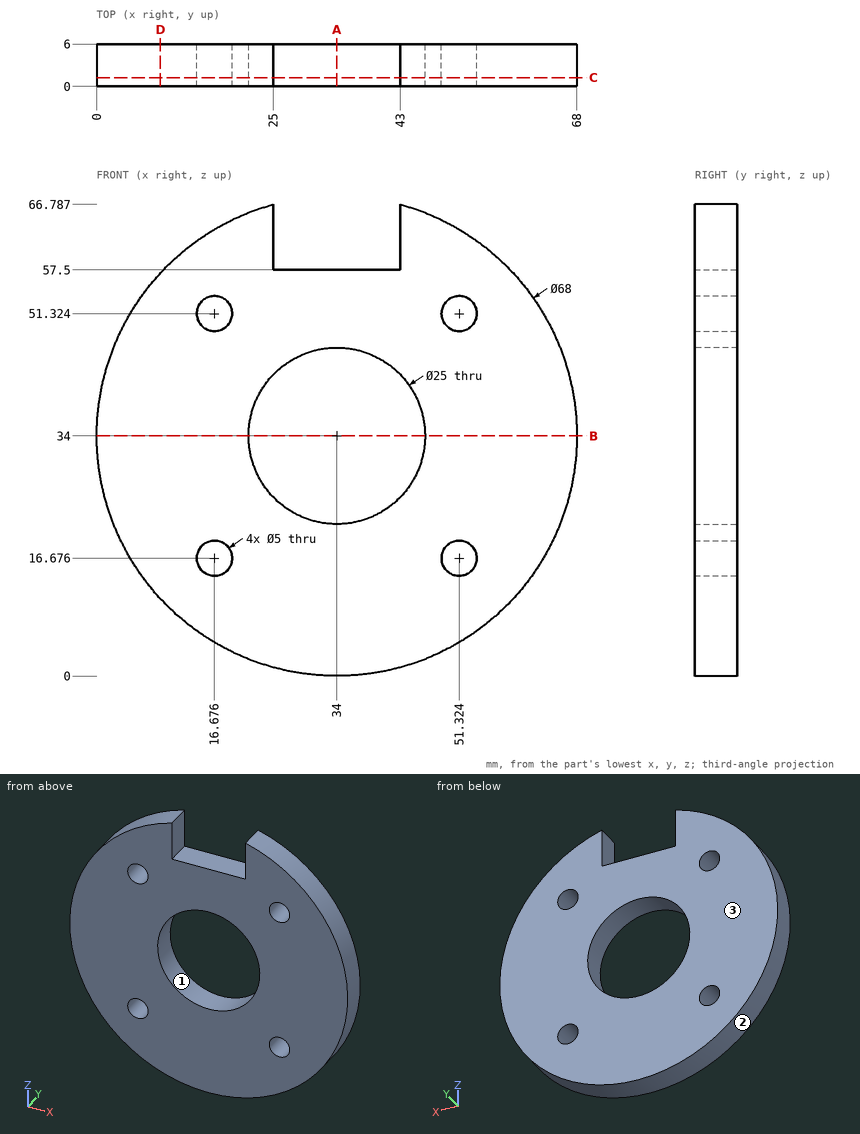
Check sheet for the drawn part. Datum: minimum x, y, z corner. Units: mm. Coordinates: 2 decimals unless noted, no trailing zeros. Order: outer loops, then holes, each group sorted by start corner. A loop starts at its lowest first (then second) coordinate and runs counter-clockwise, first axis right, second up. Notation, with made-up numbers: M 75,8 L 125,8 A10 cw 125,14 Z; hole C 9,28 d8. An arc over 180 degrees is marked long. One line per question, with ' | ' between items. Start each with the question number.
Item 1: Sectioned sample at A-A on x = 34. Record the cut outline in (y, z), and give its area (3 significant figures).
Item 2: Mould release check, pull along Z, two halves, no side actions. Record for the marked faces 1, 2 and 3: pulls with the +Z half, pulls with the -Z half, needs draft (parallel to the pull), parting line crosses it, or undercut.
Item 3: Sectioned sample at D-D on x = 9. Record the cut outline in (y, z).
Item 4: Material ranges on line 1 (Z direction, x = 18, y = 4.25) (1 decimal); line 2 (X direction, y = 2.7, z = 14.5) (1 decimal); line 3 (X direction, y = 5.4, z = 51) (1 decimal), recorded low to high.
Item 5: Sectioned sample at B-B on z = 34. Record the cut outline in (x, y).
Item 6: Gauge pin test, flat end, axial feed: P1, Ø1.8, axis at x = 35, y = 3.5, coming from the +Z side. Record the tip position at first contact, or that the pin passes through.
Item 7: Sectioned sample at C-C on y = 1.25. Record the cut outline in (x, z), and give its area (3 significant figures).
Answer below:
1) outline: M 0,0 L 6,0 L 6,21.5 L 0,21.5 Z; M 0,46.5 L 6,46.5 L 6,57.5 L 0,57.5 Z | area: 195 mm^2
2) face 1: undercut | face 2: parting line crosses it | face 3: needs draft
3) outline: M 0,10.96 L 6,10.96 L 6,57.04 L 0,57.04 Z
4) line 1: z = 4 to 14.6, 18.8 to 49.2, 53.4 to 64 | line 2: x = 6.1 to 15.4, 17.9 to 50.1, 52.6 to 61.9 | line 3: x = 4.6 to 14.2, 19.2 to 48.8, 53.8 to 63.4
5) outline: M 0,0 L 21.5,0 L 21.5,6 L 0,6 Z; M 46.5,0 L 68,0 L 68,6 L 46.5,6 Z
6) P1: stops at z = 57.5
7) outline: M 25,57.5 L 25,66.79 A34 ccw long 43,66.79 L 43,57.5 Z; hole C 16.68,16.68 d5; hole C 16.68,51.32 d5; hole C 34,34 d25; hole C 51.32,16.68 d5; hole C 51.32,51.32 d5 | area: 2,880 mm^2
